Geometry check sheet. Reference: drawing and pictorial views, mm from the part's lowest x, y, z. Coordinates: 2 decimals unless noted, no trailing zeros. Write each loop counter-clockwise with the first axis right and the second up, starting at its lowest first coordinate (ties: lowest second). Pieces come first, ordered by that corner, then holes. Notation, with made-up numbers: (35.5, 14.25) -> (46.5, 14.25) arc R26 ccw to (46.5, 46.25) -> close; hole circle Ø8 at (17.5, 75.25). An arc over 180 degrees is marked (long way). Put each result on its own line as item: value.
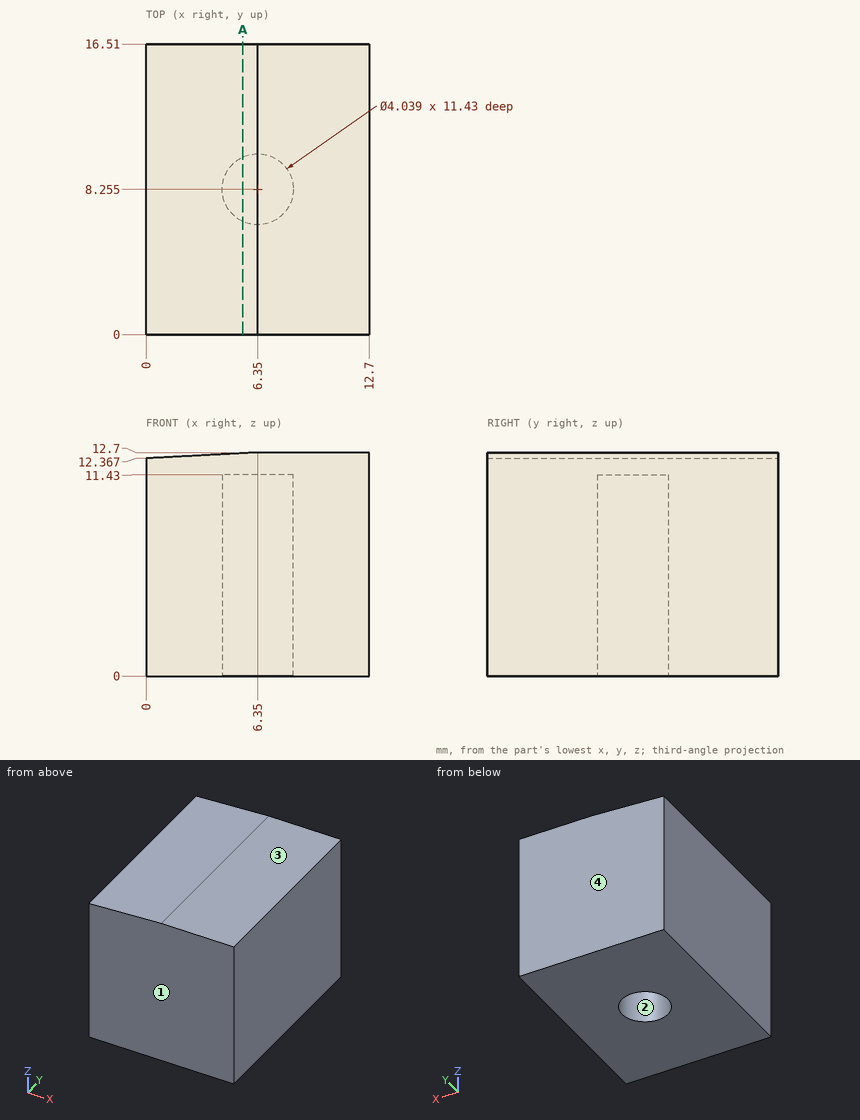
Q1. Mould release check, pull along Y, two halves, no side actions. Record for the marked faces 1, 2, 3 and 4: released by +Y, released by -Y, zero draft, split by the parting line, or undercut.
Recorded:
face 1: released by -Y
face 2: undercut
face 3: zero draft
face 4: released by +Y
Q2. Cross-section at A-A (x = 5.5). Record the cut outline in (y, z) (1 decimal), plus the area to 3 significant figures.
Recorded:
outline: (0, 0) -> (6.4, 0) -> (6.4, 11.4) -> (10.1, 11.4) -> (10.1, 0) -> (16.5, 0) -> (16.5, 12.7) -> (0, 12.7) -> close
area: 167 mm2
Q3. Depth check by flat-ended pin: P1, Ø2, axis at x = 6, y = 7.5, coming from the -Z side. Enter the tip coordinate at first touch or a pass-through.
Recorded:
P1: stops at z = 11.43
Q4. Material ranges on line 1 along Y through (x, z) = (6.35, 2.75) (1 decimal); line 2 along Z through (x, y) = (7, 7.75); line 3 along X through (y, z) = (9.25, 9.75), recorded low to high.
Recorded:
line 1: y = 0 to 6.2, 10.3 to 16.5
line 2: z = 11.43 to 12.7
line 3: x = 0 to 4.59, 8.11 to 12.7
